Part model, mm, in its own coordinate system. Coordinates: 2 decimals unless noted, no trailing zeros. Write each loop counter-clockwise with the first axis right and the second up, starting at its lowest first coordinate (ties: lowest second). Pieces come first, ordered by that corner, then holes. Notation, with made-up numbers: (-23, 25.5) -> (-8, 25.5) arc R15 ccw to (-8, 35.5) -> close; hole circle Ø4 at (36.25, 30). An arc over 180 degrees is marked (long way). One line per question, with ' | ' between items. Start each with the question number.
Item 1: Probe probe 1 along X at (y, z) = (0.2, 4.5). List the from-to ranges inside material, lowest first. Write a range as [from, to].
Item 2: Saw through at A-A (z = -37). List the corners of the cut face in (x, y), and give its area (3 significant figures).
Item 3: Pin check, flat tips, straight feed: pin 1 (3.5 mm diameter, centred on x = -62, z = 34.5, fed in from -Y); pin 2 (0.9 mm diameter, centred on x = -61, y = 2, fed in from -Z); pin 3 (1.5 mm diameter, centred on x = 61, y = 1.5, fed in from +Z). Stop position of each tip, or through.
from build123d import *

# Parameters (mm, degrees)
SKETCH1_W               = 120
SKETCH1_H               = 120
BOSS_EXTRUDE1_DEPTH     = 3.3
SKETCH2_W               = 3.3
SKETCH2_H               = 10
BOSS_EXTRUDE2_DEPTH     = 3
LPATTERN1_COUNT         = 5
LPATTERN1_PITCH         = 20
MIRROR1_COPY_1_SKETCH_W = 3.3
MIRROR1_COPY_1_SKETCH_H = 10
MIRROR1_COPY_1_DEPTH    = 3
MIRROR1_COPY_2_SKETCH_W = 3.3
MIRROR1_COPY_2_SKETCH_H = 10
MIRROR1_COPY_2_DEPTH    = 3
MIRROR1_COPY_3_SKETCH_W = 3.3
MIRROR1_COPY_3_SKETCH_H = 10
MIRROR1_COPY_3_DEPTH    = 3
MIRROR1_COPY_4_SKETCH_W = 3.3
MIRROR1_COPY_4_SKETCH_H = 10
MIRROR1_COPY_4_DEPTH    = 3


with BuildPart() as part:
    # Sketch1 → Boss-Extrude1 (new body)
    with BuildSketch(Plane(origin=(0, 0, 0), x_dir=(1, 0, 0), z_dir=(0, 1, 0))):
        Rectangle(SKETCH1_W, SKETCH1_H)
    extrude(amount=BOSS_EXTRUDE1_DEPTH)

    # Sketch2 → Boss-Extrude2 (add)
    with BuildSketch(Plane(origin=(0, 3.3, 0), x_dir=(1, 0, 0), z_dir=(0, 1, 0))):
        with Locations((61.65, 45)):
            Rectangle(SKETCH2_W, SKETCH2_H)
    boss_extrude2 = extrude(amount=-BOSS_EXTRUDE2_DEPTH)

    # LPattern1: Boss-Extrude2 ×5
    with Locations(*[(0, 0, i * LPATTERN1_PITCH) for i in range(1, LPATTERN1_COUNT)]):
        add(boss_extrude2)

    # Mirror1: Boss-Extrude2 across plane
    add(boss_extrude2.mirror(Plane(origin=(0, 0, 0), x_dir=(0, 0, 1), z_dir=(1, 0, 0))))

    # Mirror1 copy 1 sketch → Mirror1 copy 1 (add)
    with BuildSketch(Plane(origin=(0, 3.3, 20), x_dir=(-1, 0, 0), z_dir=(0, 1, 0))):
        with Locations((61.65, -45)):
            Rectangle(MIRROR1_COPY_1_SKETCH_W, MIRROR1_COPY_1_SKETCH_H)
    extrude(amount=-MIRROR1_COPY_1_DEPTH)

    # Mirror1 copy 2 sketch → Mirror1 copy 2 (add)
    with BuildSketch(Plane(origin=(0, 3.3, 40), x_dir=(-1, 0, 0), z_dir=(0, 1, 0))):
        with Locations((61.65, -45)):
            Rectangle(MIRROR1_COPY_2_SKETCH_W, MIRROR1_COPY_2_SKETCH_H)
    extrude(amount=-MIRROR1_COPY_2_DEPTH)

    # Mirror1 copy 3 sketch → Mirror1 copy 3 (add)
    with BuildSketch(Plane(origin=(0, 3.3, 60), x_dir=(-1, 0, 0), z_dir=(0, 1, 0))):
        with Locations((61.65, -45)):
            Rectangle(MIRROR1_COPY_3_SKETCH_W, MIRROR1_COPY_3_SKETCH_H)
    extrude(amount=-MIRROR1_COPY_3_DEPTH)

    # Mirror1 copy 4 sketch → Mirror1 copy 4 (add)
    with BuildSketch(Plane(origin=(0, 3.3, 80), x_dir=(-1, 0, 0), z_dir=(0, 1, 0))):
        with Locations((61.65, -45)):
            Rectangle(MIRROR1_COPY_4_SKETCH_W, MIRROR1_COPY_4_SKETCH_H)
    extrude(amount=-MIRROR1_COPY_4_DEPTH)


solid = part.part
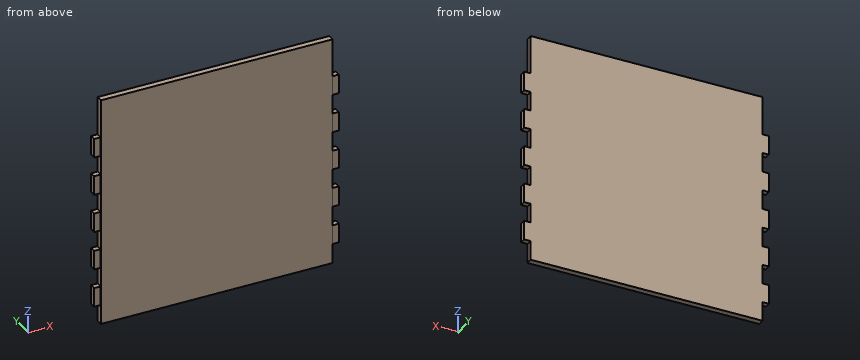
From the geometry:
1) probe 1: [-60, 60]
2) outline: (-60, 0) -> (60, 0) -> (60, 3.3) -> (-60, 3.3) -> close | area: 396 mm2
3) pin 1: y = 0.3 | pin 2: z = -50 | pin 3: z = 40
